```python
from build123d import *

# Parameters (mm, degrees)
BASE_FLANGE1_START = -3
BASE_FLANGE1_DEPTH = 3
SKETCH6_R          = 1.55
CUT_EXTRUDE1_DEPTH = 10
SKETCH7_R          = 1.55
CUT_EXTRUDE2_DEPTH = 10
SKETCH9_R          = 14.8
SKETCH9_R_2        = 13.3
SKETCH9_R_3        = 10.95
CUT_EXTRUDE4_DEPTH = 10
SKETCH8_W          = 50.2
SKETCH8_H          = 3.05
SKETCH8_W_2        = 25.1
SKETCH8_W_3        = 3.05
SKETCH8_H_2        = 15.1
CUT_EXTRUDE5_DEPTH = 10
FILLET2_R          = 0.5


# Read off the part's stored shape, not the designer's step: Base-Flange1
with BuildPart() as part:
    # Base-Flange1 outline → Base-Flange1 (new body)
    with BuildSketch(Plane(origin=(0, 0, 0), x_dir=(1, 0, 0), z_dir=(0, 1, 0)).offset(BASE_FLANGE1_START)):
        with BuildLine():
            Line((-127.928932188, 76), (127.928932188, 76))
            ThreePointArc((127.928932188, 76), (129.84234935, 76.380602337), (131.464466094, 77.464466094))
            Line((131.464466094, 77.464466094), (148.535533906, 94.535533906))
            ThreePointArc((148.535533906, 94.535533906), (149.619397663, 96.15765065), (150, 98.071067812))
            Line((150, 98.071067812), (150, 137.928932188))
            ThreePointArc((150, 137.928932188), (149.619397663, 139.84234935), (148.535533906, 141.464466094))
            Line((148.535533906, 141.464466094), (131.464466094, 158.535533906))
            ThreePointArc((131.464466094, 158.535533906), (129.84234935, 159.619397663), (127.928932188, 160))
            Line((127.928932188, 160), (-127.928932188, 160))
            ThreePointArc((-127.928932188, 160), (-129.84234935, 159.619397663), (-131.464466094, 158.535533906))
            Line((-131.464466094, 158.535533906), (-148.535533906, 141.464466094))
            ThreePointArc((-148.535533906, 141.464466094), (-149.619397663, 139.84234935), (-150, 137.928932188))
            Line((-150, 137.928932188), (-150, 98.071067812))
            ThreePointArc((-150, 98.071067812), (-149.619397663, 96.15765065), (-148.535533906, 94.535533906))
            Line((-148.535533906, 94.535533906), (-131.464466094, 77.464466094))
            ThreePointArc((-131.464466094, 77.464466094), (-129.84234935, 76.380602337), (-127.928932188, 76))
        make_face()
    extrude(amount=BASE_FLANGE1_DEPTH)

    # Sketch6 → Cut-Extrude1 (cut)
    with BuildSketch(Plane(origin=(0, 0, 0), x_dir=(1, 0, 0), z_dir=(0, 1, 0))):
        with Locations(Location((128, 146, 0), (0, 0, 270))):
            Circle(SKETCH6_R)
        with Locations(Location((-128, 146, 0), (0, 0, 90))):
            Circle(SKETCH6_R)
    extrude(amount=-CUT_EXTRUDE1_DEPTH, mode=Mode.SUBTRACT)

    # Sketch7 → Cut-Extrude2 (cut)
    with BuildSketch(Plane(origin=(0, 0, 0), x_dir=(1, 0, 0), z_dir=(0, 1, 0))):
        with Locations(Location((-128, 94, 0), (0, 0, 270))):
            Circle(SKETCH7_R)
        with Locations(Location((128, 94, 0), (0, 0, 90))):
            Circle(SKETCH7_R)
    extrude(amount=-CUT_EXTRUDE2_DEPTH, mode=Mode.SUBTRACT)

    # Sketch9 → Cut-Extrude4 (cut)
    with BuildSketch(Plane(origin=(0, 0, 0), x_dir=(1, 0, 0), z_dir=(0, 1, 0))):
        with Locations(Location((-65.3, 118, 0), (0, 0, 270))):
            Circle(SKETCH9_R)
        with Locations(Location((65.3, 118, 0), (0, 0, 270))):
            Circle(SKETCH9_R)
        with Locations(Location((-107.3, 118, 0), (0, 0, 270))):
            Circle(SKETCH9_R_2)
        with Locations(Location((107.3, 118, 0), (0, 0, 270))):
            Circle(SKETCH9_R_3)
        with BuildLine():
            Line((-32.9, 83.9), (32.9, 83.9))
            ThreePointArc((32.9, 83.9), (33.182842712, 84.017157288), (33.3, 84.3))
            Line((33.3, 84.3), (33.3, 110.2))
            ThreePointArc((33.3, 110.2), (33.182842712, 110.482842712), (32.9, 110.6))
            Line((32.9, 110.6), (26.3, 110.6))
            ThreePointArc((26.3, 110.6), (25.592893219, 110.892893219), (25.3, 111.6))
            Line((25.3, 111.6), (25.3, 122.8))
            ThreePointArc((25.3, 122.8), (25.592893219, 123.507106781), (26.3, 123.8))
            Line((26.3, 123.8), (32.9, 123.8))
            ThreePointArc((32.9, 123.8), (33.182842712, 123.917157288), (33.3, 124.2))
            Line((33.3, 124.2), (33.3, 150.1))
            ThreePointArc((33.3, 150.1), (33.182842712, 150.382842712), (32.9, 150.5))
            Line((32.9, 150.5), (-32.9, 150.5))
            ThreePointArc((-32.9, 150.5), (-33.182842712, 150.382842712), (-33.3, 150.1))
            Line((-33.3, 150.1), (-33.3, 124.2))
            ThreePointArc((-33.3, 124.2), (-33.182842712, 123.917157288), (-32.9, 123.8))
            Line((-32.9, 123.8), (-26.3, 123.8))
            ThreePointArc((-26.3, 123.8), (-25.592893219, 123.507106781), (-25.3, 122.8))
            Line((-25.3, 122.8), (-25.3, 111.6))
            ThreePointArc((-25.3, 111.6), (-25.592893219, 110.892893219), (-26.3, 110.6))
            Line((-26.3, 110.6), (-32.9, 110.6))
            ThreePointArc((-32.9, 110.6), (-33.182842712, 110.482842712), (-33.3, 110.2))
            Line((-33.3, 110.2), (-33.3, 84.3))
            ThreePointArc((-33.3, 84.3), (-33.182842712, 84.017157288), (-32.9, 83.9))
        make_face()
        with BuildLine():
            Line((-28.25, 119.2), (-28.25, 115.2))
            ThreePointArc((-28.25, 115.2), (-30.3, 113.15), (-32.35, 115.2))
            Line((-32.35, 115.2), (-32.35, 119.2))
            ThreePointArc((-32.35, 119.2), (-30.3, 121.25), (-28.25, 119.2))
        make_face()
        with BuildLine():
            Line((28.25, 119.2), (28.25, 115.2))
            ThreePointArc((28.25, 115.2), (30.3, 113.15), (32.35, 115.2))
            Line((32.35, 115.2), (32.35, 119.2))
            ThreePointArc((32.35, 119.2), (30.3, 121.25), (28.25, 119.2))
        make_face()
    extrude(amount=-CUT_EXTRUDE4_DEPTH, mode=Mode.SUBTRACT)

    # Sketch8 → Cut-Extrude5 (cut)
    with BuildSketch(Plane(origin=(0, 0, 0), x_dir=(1, 0, 0), z_dir=(0, 1, 0))):
        with Locations((0, 82.375)):
            Rectangle(SKETCH8_W, SKETCH8_H)
        with Locations((87.45, 82.375)):
            Rectangle(SKETCH8_W_2, SKETCH8_H)
        with Locations((136.475, 132.45)):
            Rectangle(SKETCH8_W_3, SKETCH8_H_2)
        with Locations((0, 152.025)):
            Rectangle(SKETCH8_W, SKETCH8_H)
        with Locations((87.45, 152.025)):
            Rectangle(SKETCH8_W_2, SKETCH8_H)
        with Locations((-87.45, 152.025)):
            Rectangle(SKETCH8_W_2, SKETCH8_H)
        with Locations((136.475, 101.55)):
            Rectangle(SKETCH8_W_3, SKETCH8_H_2)
        with Locations((-87.45, 82.375)):
            Rectangle(SKETCH8_W_2, SKETCH8_H)
        with Locations((-136.475, 101.55)):
            Rectangle(SKETCH8_W_3, SKETCH8_H_2)
        with Locations((-136.475, 132.45)):
            Rectangle(SKETCH8_W_3, SKETCH8_H_2)
    extrude(amount=-CUT_EXTRUDE5_DEPTH, mode=Mode.SUBTRACT)

    # Fillet2
    fillet2_edges = [part.edges().sort_by_distance(p)[0] for p in [
        (-25.1, -1.5, -150.5),
        (25.1, -1.5, -150.5),
        (-25.1, -1.5, -83.9),
        (25.1, -1.5, -83.9),
    ]]
    fillet(fillet2_edges, radius=FILLET2_R)


solid = part.part
```
Geometry check sheet. Reference: the model listing, model coordinates, mm. Round coordinates to 2 decimals unless told otherwise and drop trailing zeros. Loops run counter-clockwise (first coordinate to the right, second up) from the corner with the lowest first, then second, coordinate; pieces in that order, holes last. Notation, with made-up numbers: (-14.75, 71.25) - (8.25, 71.25) arc R24 ccw to (8.25, 99.25) - close; hole circle Ø9 at (-37, -13). An arc over 180 degrees is marked (long way). Use a Markdown table: item, result.
Q1. Draft check along X on faces 1 (the flat face through (140, -2, -86)), 2 (the cylindrical face through (-60.854, -1.479, -103.883)), 3 (the flat face through (-140, -2, -150)). Enter one of: released by +X, released by -X, zero draft, split by the parting line, or undercut.
Solutions:
| item | result |
|---|---|
| face 1 | released by +X |
| face 2 | undercut |
| face 3 | released by -X |
Q2. Go/stop test with flat-tipped pins: P1, Ø4, axis at x = 128, z = -146, coming from the +Y side; P2, Ø1.5, axis at y = -1, z = -152, coming from the -X side; P3, Ø1.5, axis at y = -0.5, z = -144, coming from the +X side; P4, Ø0.9, axis at x = -136.5, y = -1, coming from the +Z side. Record where each tip stops, or that it passes through.
Solutions:
| item | result |
|---|---|
| P1 | stops at y = 0 |
| P2 | stops at x = -138.75 |
| P3 | stops at x = 146.75 |
| P4 | stops at z = -82.05 |
Q3. Cross-section at C-C on y = -0.95. State how many separate pieces and enclosed holes the cut face has, plus the area to 3 significant figures.
Solutions:
| item | result |
|---|---|
| separate pieces | 1 |
| enclosed holes | 19 |
| area | 17,000 mm2 |
Q4. Cross-section at B-B on x = -17.5. Record the cut outline in (y, z), plus the area to 3 significant figures.
Solutions:
| item | result |
|---|---|
| outline | (-3, -160) - (0, -160) - (0, -153.55) - (-3, -153.55) - close; (-3, -80.85) - (0, -80.85) - (0, -76) - (-3, -76) - close |
| area | 33.9 mm2 |
Q5. Material ranges on line 1 (Z direction, x = -27, y = -0.55); line 2 (X direction, y = -0.9, z = -100); line 3 (Z direction, x = 128, y = -1.7), recorded low to high.
Solutions:
| item | result |
|---|---|
| line 1 | z = -160 to -150.5, -123.8 to -110.6, -83.9 to -76 |
| line 2 | x = -150 to -138, -134.95 to -33.3, 33.3 to 134.95, 138 to 150 |
| line 3 | z = -160 to -147.55, -144.45 to -95.55, -92.45 to -76 |
Q6. Cross-section at A-A on x = 65.3. Record the cut outline in (y, z).
Solutions:
| item | result |
|---|---|
| outline | (-3, -160) - (0, -160) - (0, -132.8) - (-3, -132.8) - close; (-3, -103.2) - (0, -103.2) - (0, -76) - (-3, -76) - close |
